from build123d import *

# Parameters (mm, degrees)
SKETCH1_W           = 54
SKETCH1_H           = 65
BOSS_EXTRUDE1_DEPTH = 10
SKETCH2_W           = 20
SKETCH2_H           = 30
BOSS_EXTRUDE2_DEPTH = 30
FILLET1_R           = 15
SKETCH3_R           = 11
CUT_EXTRUDE1_DEPTH  = 7
SKETCH4_R           = 6
CUT_EXTRUDE2_DEPTH  = 5
SKETCH5_R           = 1.5875
CUT_EXTRUDE3_DEPTH  = 7
SKETCH6_R           = 2.3241
CUT_EXTRUDE4_DEPTH  = 6


with BuildPart() as part:
    # Sketch1 → Boss-Extrude1 (new body)
    with BuildSketch(Plane(origin=(0, 0, 0), x_dir=(1, 0, 0), z_dir=(0, 1, 0))):
        Rectangle(SKETCH1_W, SKETCH1_H)
    extrude(amount=BOSS_EXTRUDE1_DEPTH)

    # Sketch2 → Boss-Extrude2 (add)
    with BuildSketch(Plane.XZ):
        with Locations((7, 0)):
            Rectangle(SKETCH2_W, SKETCH2_H)
    extrude(amount=BOSS_EXTRUDE2_DEPTH)

    # Fillet1
    fillet1_edges = [part.edges().sort_by_distance(p)[0] for p in [
        (7, -30, -15),
        (7, -30, 15),
    ]]
    fillet(fillet1_edges, radius=FILLET1_R - 0.0001)  # a hair under: the kernel refuses the full size

    # Sketch3 → Cut-Extrude1 (cut)
    with BuildSketch(Plane(origin=(17, 0, 0), x_dir=(0, 0, -1), z_dir=(1, 0, 0))):
        with Locations((0, -15)):
            Circle(SKETCH3_R)
    extrude(amount=-CUT_EXTRUDE1_DEPTH, mode=Mode.SUBTRACT)

    # Sketch4 → Cut-Extrude2 (cut)
    with BuildSketch(Plane.ZY.offset(3)):
        with Locations((0, -15)):
            Circle(SKETCH4_R)
    extrude(amount=-CUT_EXTRUDE2_DEPTH, mode=Mode.SUBTRACT)

    # Sketch5 → Cut-Extrude3 (cut)
    with BuildSketch(Plane.ZY.offset(3)):
        with Locations((0, -5.5)):
            Circle(SKETCH5_R)
        with Locations((8.227241336, -10.25)):
            Circle(SKETCH5_R)
        with Locations((8.227241336, -19.75)):
            Circle(SKETCH5_R)
        with Locations((0, -24.5)):
            Circle(SKETCH5_R)
        with Locations((-8.227241336, -19.75)):
            Circle(SKETCH5_R)
        with Locations((-8.227241336, -10.25)):
            Circle(SKETCH5_R)
    extrude(amount=-CUT_EXTRUDE3_DEPTH, mode=Mode.SUBTRACT)

    # Sketch6 → Cut-Extrude4 (cut)
    with BuildSketch(Plane(origin=(10, 0, 0), x_dir=(0, 0, -1), z_dir=(1, 0, 0))):
        with Locations((0, -5.5)):
            Circle(SKETCH6_R)
        with Locations((8.227241336, -10.25)):
            Circle(SKETCH6_R)
        with Locations((8.227241336, -19.75)):
            Circle(SKETCH6_R)
        with Locations((0, -24.5)):
            Circle(SKETCH6_R)
        with Locations((-8.227241336, -19.75)):
            Circle(SKETCH6_R)
        with Locations((-8.227241336, -10.25)):
            Circle(SKETCH6_R)
    extrude(amount=-CUT_EXTRUDE4_DEPTH, mode=Mode.SUBTRACT)


solid = part.part
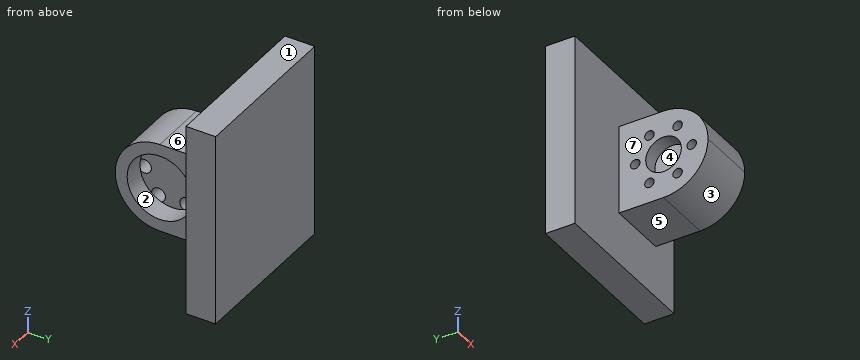
Can you work these out from the model? Positions are in its coordinate system, mm. Face numbers are marked on the shaded views. A direction names the side the tool comes from. Round coordinates to 2 decimals unless told otherwise and drop trailing zeros. Write each loop counter-clockwise with the first axis right and the second up, starting at its lowest first coordinate (ties: lowest second). Pieces come first, ordered by that corner, then holes. Notation, with made-up numbers: (-39.5, -40) - (-34.5, -40) arc R26 cw to (-34.5, -10) - close; hole circle Ø11 at (-25, -1.75). An arc over 180 degrees is marked (long way). Write each question's results on one line, items separated by ' | '. Start each with the question number.
1) We'd pull the mould along Z, two halves only. Please class the marked faces 1, 2, 3 and 4: released by +Z, released by -Z, zero draft, split by the parting line, or undercut.
2) Suppose I cut it at B-B (z = 7.5). List the corners of the cut face in (x, y) for me, and give its area (3 significant figures).
3) For pin 1 Ø0.5 at (y, z) = (-3.5, 0.5) entering from -X; pin 2 Ø1.4 at (y, z) = (-21, 9) entering from +X; pin 3 Ø7 at (y, z) = (-15, 0) entering from -X, each with a flat end and sliding along its axis, tell me the tip position at first contact or that it passes through.
4) Which directions (+Z, -Z, +X, -X, +Y, -Y) give clear straight access to the entire face, cutting with the end or side of a thin tool? Please do the marked faces 5, 6 and 7.
5) Please list where these lines run through material, in increasing order: line 1 (Y direction, x = 15, z = 0); line 2 (X direction, y = -4, z = -1); line 3 (Y direction, x = 8.5, z = -18).
6) Suppose I cut it at A-A (x = 5). Give the number of separate pieces and of enclosed holes in the cut face, and give its area (3 significant figures).
7) Suppose I cut it at D-D (y = -19.75). List the corners of the cut face in (x, z) for me.
8) Suppose I cut it at C-C (y = -24.5). List the corners of the cut face in (x, z) for me.
Here are the results:
1) face 1: released by +Z | face 2: undercut | face 3: released by -Z | face 4: undercut
2) outline: (-27, 0) - (-3, 0) - (-3, -8.84) - (4, -8.84) - (4, -8.04) - (10, -8.04) - (10, -6.95) - (17, -6.95) - (17, 0) - (27, 0) - (27, 10) - (-27, 10) - close; (-3, -27.99) - (17, -27.99) - (17, -23.05) - (10, -23.05) - (10, -21.96) - (4, -21.96) - (4, -21.16) - (-3, -21.16) - close; (-3, -18.34) - (4, -18.34) - (4, -17.54) - (10, -17.54) - (10, -12.46) - (4, -12.46) - (4, -11.66) - (-3, -11.66) - close | area: 895 mm2
3) pin 1: stops at x = -3 | pin 2: stops at x = 17 | pin 3: stops at x = 2
4) face 5: -Z, +X, -X, -Y | face 6: +Z, +X, -X, -Y | face 7: +Z, -Z, -X, -Y
5) line 1: y = -30 to -26, -4 to 10 | line 2: x = -3 to 4, 10 to 17 | line 3: y = 0 to 10
6) separate pieces: 1 | enclosed holes: 6 | area: 1,350 mm2
7) outline: (-3, -14.23) - (17, -14.23) - (17, -9.92) - (10, -9.92) - (10, -10.55) - (4, -10.55) - (4, -9.81) - (-3, -9.81) - close; (-3, -6.64) - (4, -6.64) - (4, -5.9) - (10, -5.9) - (10, 5.9) - (4, 5.9) - (4, 6.64) - (-3, 6.64) - (-3, 3.67) - (2, 3.67) - (2, -3.67) - (-3, -3.67) - close; (-3, 9.81) - (4, 9.81) - (4, 10.55) - (10, 10.55) - (10, 9.92) - (17, 9.92) - (17, 14.23) - (-3, 14.23) - close
8) outline: (-3, -11.61) - (17, -11.61) - (17, -5.55) - (10, -5.55) - (10, -2.32) - (4, -2.32) - (4, -1.59) - (-3, -1.59) - close; (-3, 1.59) - (4, 1.59) - (4, 2.32) - (10, 2.32) - (10, 5.55) - (17, 5.55) - (17, 11.61) - (-3, 11.61) - close
